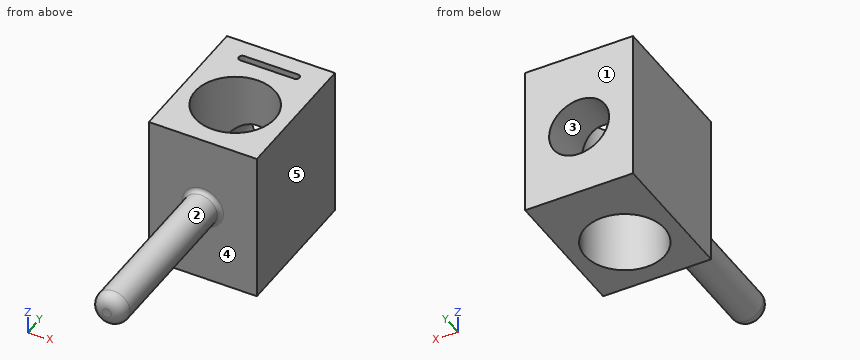
from build123d import *

# Parameters (mm, degrees)
SKETCH_1_W           = 2.7
SKETCH_1_H           = 3.5
EXTRUDE_1_DEPTH      = 3.8
SKETCH_2_OUTSIDE_W   = 5.866
SKETCH_2_OUTSIDE_H   = 6.666
SKETCH_2_OUTSIDE_W_2 = 2.7
SKETCH_2_OUTSIDE_H_2 = 3.5
SKETCH_2_OUTSIDE_R   = 1
CUT_EXTRUDE_1_DEPTH  = 5.396020928
SKETCH_4_OUTSIDE_W   = 5.866
SKETCH_4_OUTSIDE_H   = 6.966
SKETCH_4_OUTSIDE_W_2 = 2.7
SKETCH_4_OUTSIDE_H_2 = 3.8
SKETCH_4_OUTSIDE_R   = 0.75
CUT_EXTRUDE_2_DEPTH  = 1.85
CUT_EXTRUDE_3_DEPTH  = 0.5
SKETCH_6_R           = 0.415
EXTRUDE_2_DEPTH      = 4.31
FILLET_1_R           = 0.3
FILLET_2_R           = 0.1


with BuildPart() as part:
    # Эскиз1 → Бобышка-Вытянуть1 (new body)
    with BuildSketch(Plane.XY):
        Rectangle(SKETCH_1_W, SKETCH_1_H)
    extrude(amount=-EXTRUDE_1_DEPTH)

    # Эскиз2 outside → Вырез-Вытянуть1 (cut, through all)
    # profile 1 of 2: a face of its own
    with BuildSketch(Plane.XY):
        Rectangle(SKETCH_2_OUTSIDE_W, SKETCH_2_OUTSIDE_H)
        Rectangle(SKETCH_2_OUTSIDE_W_2, SKETCH_2_OUTSIDE_H_2, mode=Mode.SUBTRACT)
    # profile 2 of 2: a face of its own
    with BuildSketch(Plane.XY):
        with Locations((0, -0.3)):
            Circle(SKETCH_2_OUTSIDE_R)
    extrude(amount=-CUT_EXTRUDE_1_DEPTH, mode=Mode.SUBTRACT)

    # Эскиз4 outside → Вырез-Вытянуть2 (cut)
    # profile 1 of 2: a face of its own
    with BuildSketch(Plane(origin=(0, 1.75, 0), x_dir=(1, 0, 0), z_dir=(0, 1, 0))):
        with Locations((0, 1.9)):
            Rectangle(SKETCH_4_OUTSIDE_W, SKETCH_4_OUTSIDE_H)
        with Locations((0, 1.9)):
            Rectangle(SKETCH_4_OUTSIDE_W_2, SKETCH_4_OUTSIDE_H_2, mode=Mode.SUBTRACT)
    # profile 2 of 2: a face of its own
    with BuildSketch(Plane(origin=(0, 1.75, 0), x_dir=(1, 0, 0), z_dir=(0, 1, 0))):
        with Locations(Location((0, 2, 0), (0, 0, 270))):
            Circle(SKETCH_4_OUTSIDE_R)
    extrude(amount=-CUT_EXTRUDE_2_DEPTH, mode=Mode.SUBTRACT)

    # Эскиз5 → Вырез-Вытянуть3 (cut)
    with BuildSketch(Plane.XY):
        with BuildLine():
            Line((-0.675, 1.311413609), (0.675, 1.311413609))
            ThreePointArc((0.675, 1.311413609), (0.761413609, 1.225), (0.675, 1.138586391))
            Line((0.675, 1.138586391), (-0.675, 1.138586391))
            ThreePointArc((-0.675, 1.138586391), (-0.761413609, 1.225), (-0.675, 1.311413609))
        make_face()
    extrude(amount=-CUT_EXTRUDE_3_DEPTH, mode=Mode.SUBTRACT)

    # Эскиз6 → Бобышка-Вытянуть2 (add)
    with BuildSketch(Plane.XZ.offset(1.75)):
        with Locations(Location((0, -1.85, 0), (0, 0, 270))):
            Circle(SKETCH_6_R)
    extrude(amount=EXTRUDE_2_DEPTH)

    # Скругление1
    fillet_1_edges = [part.edges().sort_by_distance(p)[0] for p in [
        (0, -6.06, -1.435),
    ]]
    fillet(fillet_1_edges, radius=FILLET_1_R)

    # Скругление2
    fillet_2_edges = [part.edges().sort_by_distance(p)[0] for p in [
        (0, -1.75, -1.435),
    ]]
    fillet(fillet_2_edges, radius=FILLET_2_R)


solid = part.part
Check sheet for the modelled part. Datum: model origin and axes. Units: mm. Face numbers are marked on the shaded views. A direction names the side the tool comes from. Round coordinates to 2 decimals unless told otherwise and drop trailing zeros. Loops run counter-clockwise (first coordinate to the right, second up) from the corner with the lowest first, then second, coordinate; pieces in that order, holes last. Notation, with made-up numbers: M 38,79.25 L 72,79.25 A24 cw 72,92.25 Z; hole C 23,54 d11. An arc over 180 degrees is marked long. One line per question, with ' | ' between items. Start each with the question number.
Item 1: Section check A-A (x = 0.6). Record the boundary of the cut face in (y, z), and give its area (3 significant figures).
Item 2: Section check C-C (y = 1). Record the boundary of the cut face in (x, z).
Item 3: Gauge pin test, flat ends, axial feed: pin 1 Ø0.8 at (x, z) = (0, -2.5) entering from -Y; pin 2 Ø1 at (x, y) = (0, -4) entering from -Z (3 decimals). Record the tip position at first contact, or that the pin passes through.
Item 4: Section check B-B (y = -0.3). Record the boundary of the cut face in (x, z).
Item 5: Section check D-D (z = -2.85). Record the boundary of the cut face in (x, y).
Item 6: Scan lines: probe 1 along Y at (x, z) = (0, -3); probe 2 along X at (y, z) = (0.9, -2); probe 3 along Z at (x, y) = (0, 1.1). Record each from-to range of solid material in increasing order.
Item 7: Set-up check for the marked faces 4 and 5: record each of +Z, -Z, +X, -X, +Y, -Y from which the full face is reachable in a straight line by a thin tool's end or side.
Item 8: Release check for a two-part mould opening along Z. For the marked faces 1, 2 and 3 record: released by +Z, released by -Z, zero draft, split by the parting line, or undercut.
Worked out:
1) outline: M -1.75,-3.8 L -1.1,-3.8 L -1.1,0 L -1.75,0 Z; M 0.5,-3.8 L 1.75,-3.8 L 1.75,-2.45 L 0.5,-2.45 Z; M 0.5,-1.55 L 1.75,-1.55 L 1.75,0 L 1.31,0 L 1.31,-0.5 L 1.14,-0.5 L 1.14,0 L 0.5,0 Z | area: 6.01 mm^2
2) outline: M -1.35,-3.8 L 1.35,-3.8 L 1.35,0 L -1.35,0 Z; hole C 0,-2 d1.5
3) pin 1: y = -6.03 | pin 2: z = -2.265
4) outline: M -1.35,-3.8 L -1,-3.8 L -1,0 L -1.35,0 Z; M 1,-3.8 L 1.35,-3.8 L 1.35,0 L 1,0 Z
5) outline: M -1.35,-1.75 L 1.35,-1.75 L 1.35,1.75 L -1.35,1.75 Z; hole C 0,-0.3 d2
6) probe 1: -1.75 to -1.3, 0.7 to 1.75 | probe 2: -1.35 to -0.75, 0.75 to 1.35 | probe 3: -3.8 to -2.75, -1.25 to 0
7) face 4: -Y | face 5: +Z, -Z, +X, +Y, -Y
8) face 1: zero draft | face 2: split by the parting line | face 3: undercut
